Can you work these out from the model? Positions are in its coordinate system, mm. Face numbers are marked on the shaded views. A direction names the side the tool comes from. Round coordinates to 2 decimals unless told otherwise and drop trailing zeros. Order: outer loops, then holes, each group sorted by start corner. A loop starts at its lowest first (then second) coordinate and runs counter-clockwise, first axis right, second up.
Q1. If we section it at B-B (y = 1): Please give me the cut outline in (x, z), plus the area to 3 significant figures.
Q2. If we section it at C-C (x = 57): Please give me the cut outline in (y, z).
Q3. We'd pull the mould along X, two halves only. Please class the marked faces 3, 4 and 5: pulls with the +X half, pulls with the -X half, needs draft (parallel to the pull), parting line crosses it, or undercut.
Q4. If we section it at A-A (y = 5.75): Please give me the cut outline in (x, z).
Q5. If I drill on line 1 (Y direction, x = 42, z = -17); line 2 (Z direction, x = 79.5, y = 2.25); line 3 (Z direction, x = 78, y = 3.75), over which ranges is the centre line in solid material (lowest first)?
Q6. Will these pins go through, and if not, where does the flat tip stop? P1, Ø8, axis at x = 28, z = -19, coming from the +Y side; P2, Ø2, axis at y = 5.5, z = 1.5, coming from the +X side; P3, Ø6, axis at x = 12.5, z = -2.5, coming from the -Y side.
Q7. If we section it at D-D (z = -23): Please give me the cut outline in (x, y).
Q8. For the marked faces 1 and 2, which set-ups out of +Z, -Z, +X, -X, +Y, -Y let a thin tool reach every point of the face, with its end or its side?
from build123d import *

# Parameters (mm, degrees)
SKETCH1_R           = 2.25
BOSS_EXTRUDE1_DEPTH = 3
SKETCH6_R           = 2.25
BOSS_EXTRUDE3_DEPTH = 4.5
BOSS_EXTRUDE4_START = -3
SKETCH6_4_R         = 2.25
BOSS_EXTRUDE4_DEPTH = 4.5


with BuildPart() as part:
    # Sketch1 → Boss-Extrude1 (new body)
    with BuildSketch(Plane(origin=(0, 0, 0), x_dir=(1, 0, 0), z_dir=(0, 1, 0))):
        with BuildLine():
            Line((4.346556407, 16.19061741), (0, 0))
            Line((0, 0), (21.097139824, 0))
            Line((21.097139824, 0), (23.621877097, 9.40446906))
            Line((23.621877097, 9.40446906), (55.315636071, 0.895916999))
            Line((55.315636071, 0.895916999), (63.837679632, -8.03903216))
            ThreePointArc((63.837679632, -8.03903216), (66.877486097, -9.287511543), (69.837996716, -7.861152194))
            Line((69.837996716, -7.861152194), (72.354139199, -4.888856081))
            ThreePointArc((72.354139199, -4.888856081), (85.255098096, -4.502096268), (86.353286495, 8.357853416))
            Line((86.353286495, 8.357853416), (89.383500932, 10.135016952))
            ThreePointArc((89.383500932, 10.135016952), (80.259194518, 15.628469331), (70.012090644, 12.72539359))
            Line((70.012090644, 12.72539359), (20.281795984, 26.10351195))
            ThreePointArc((20.281795984, 26.10351195), (10.910267874, 25.037898105), (4.794128684, 17.857792715))
            Line((4.794128684, 17.857792715), (4.346556407, 16.19061741))
        make_face()
        with Locations((78.484447615, 2.356518872)):
            Circle(SKETCH1_R, mode=Mode.SUBTRACT)
        with Locations((38.137547341, 13.414423288)):
            Circle(SKETCH1_R, mode=Mode.SUBTRACT)
    extrude(amount=BOSS_EXTRUDE1_DEPTH)

    # Sketch6 → Boss-Extrude3 (add)
    with BuildSketch(Plane(origin=(0, 3, 0), x_dir=(1, 0, 0), z_dir=(0, 1, 0))):
        with BuildLine():
            Line((46.466786902, 3.271491758), (55.315636071, 0.895916999))
            Line((55.315636071, 0.895916999), (63.837679632, -8.03903216))
            ThreePointArc((63.837679632, -8.03903216), (66.877486097, -9.287511543), (69.837996716, -7.861152194))
            Line((69.837996716, -7.861152194), (72.354139199, -4.888856081))
            ThreePointArc((72.354139199, -4.888856081), (85.255098096, -4.502096268), (86.353286495, 8.357853416))
            Line((86.353286495, 8.357853416), (89.383500932, 10.135016952))
            ThreePointArc((89.383500932, 10.135016952), (80.259194518, 15.628469331), (70.012090644, 12.72539359))
            Line((70.012090644, 12.72539359), (50.427328439, 17.993958126))
            Line((50.427328439, 17.993958126), (46.466786902, 3.271491758))
        make_face()
        with Locations((78.484447615, 2.356518872)):
            Circle(SKETCH6_R, mode=Mode.SUBTRACT)
    extrude(amount=BOSS_EXTRUDE3_DEPTH)

    # Sketch6<4> → Boss-Extrude4 (add)
    with BuildSketch(Plane(origin=(0, 3, 0), x_dir=(1, 0, 0), z_dir=(0, 1, 0)).offset(BOSS_EXTRUDE4_START)):
        with BuildLine():
            Line((46.466786902, 3.271491758), (55.315636071, 0.895916999))
            Line((55.315636071, 0.895916999), (63.837679632, -8.03903216))
            ThreePointArc((63.837679632, -8.03903216), (66.877486097, -9.287511543), (69.837996716, -7.861152194))
            Line((69.837996716, -7.861152194), (72.354139199, -4.888856081))
            ThreePointArc((72.354139199, -4.888856081), (85.255098096, -4.502096268), (86.353286495, 8.357853416))
            Line((86.353286495, 8.357853416), (89.383500932, 10.135016952))
            ThreePointArc((89.383500932, 10.135016952), (80.259194518, 15.628469331), (70.012090644, 12.72539359))
            Line((70.012090644, 12.72539359), (50.427328439, 17.993958126))
            Line((50.427328439, 17.993958126), (46.466786902, 3.271491758))
        make_face()
        with Locations((78.484447615, 2.356518872)):
            Circle(SKETCH6_4_R, mode=Mode.SUBTRACT)
    extrude(amount=-BOSS_EXTRUDE4_DEPTH)


solid = part.part
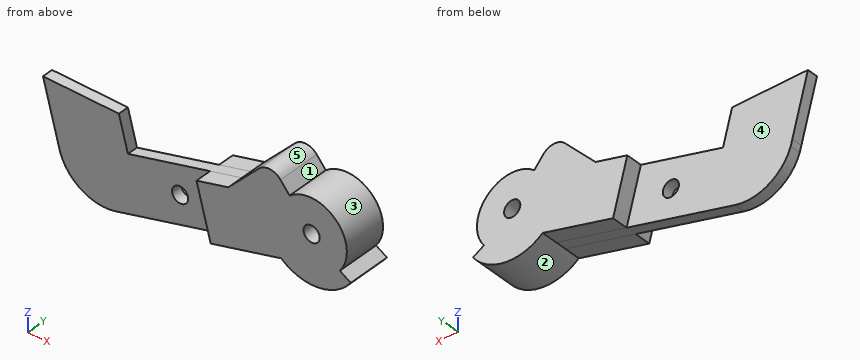
Solution:
1. outline: (0, 0) - (4.79, -17.86) arc R12.84 ccw to (20.28, -26.1) - (70.01, -12.73) arc R13.39 ccw to (89.38, -10.14) - (86.35, -8.36) arc R9.7 ccw to (72.35, 4.89) - (69.84, 7.86) arc R4.04 ccw to (63.84, 8.04) - (55.32, -0.9) - (23.62, -9.4) - (21.1, 0) - close; hole circle Ø4.5 at (38.14, -13.41); hole circle Ø4.5 at (78.48, -2.36)
1. area: 1,640 mm2
2. outline: (-4.5, -16.23) - (7.5, -16.23) - (7.5, 0.87) - (-4.5, 0.87) - close
3. face 3: undercut
3. face 4: needs draft
3. face 5: parting line crosses it
4. outline: (46.47, -3.27) - (50.43, -17.99) - (70.01, -12.73) arc R13.39 ccw to (89.38, -10.14) - (86.35, -8.36) arc R9.7 ccw to (72.35, 4.89) - (69.84, 7.86) arc R4.04 ccw to (63.84, 8.04) - (55.32, -0.9) - close; hole circle Ø4.5 at (78.48, -2.36)
5. line 1: y = 0 to 3
5. line 2: z = -15.71 to -4.36, -0.35 to 7.11
5. line 3: z = -15.74 to -4.55, -0.16 to 7.14
6. P1: stops at y = 3
6. P2: stops at x = 87.8
6. P3: stops at y = 0
7. outline: (8.09, 0) - (31.82, 0) - (31.82, 3) - (8.09, 3) - close
8. face 1: +Z, +Y, -Y
8. face 2: -Z, +Y, -Y
